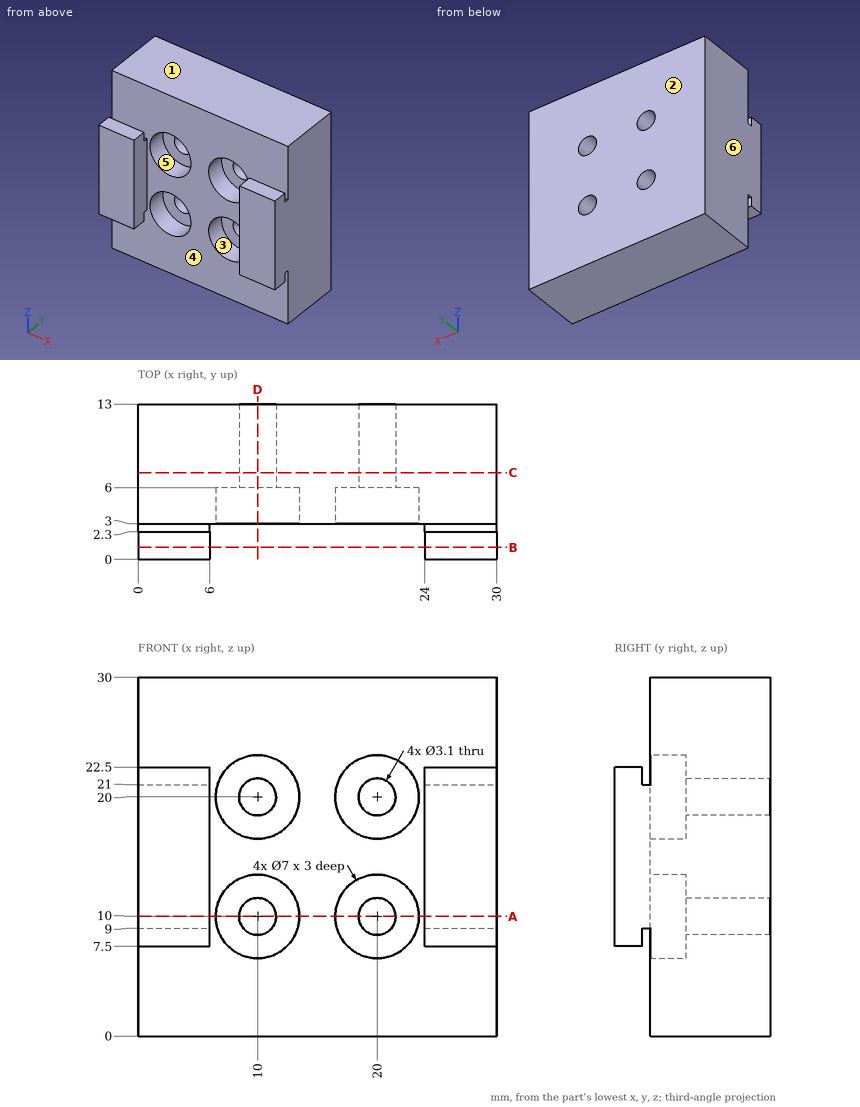
Answer from the drawing. Dimensions are ordinates in mm from the lowest x, y and z of the part. A direction names the side the tool comes from. Give positions to 0.01 mm unless a question says otherwise; leave off trailing zeros. Write each loop counter-clockwise with the first axis right and the second up, starting at its lowest first coordinate (ties: lowest second). Pieces come first, ordered by that corner, then holes. Notation, with made-up numbers: (78.5, 25.5) -> (85.5, 25.5) arc R9 ccw to (85.5, 30.5) -> close; hole circle Ø10 at (28, -18.75). An arc over 180 degrees is marked (long way). One line per question, with ' | ' between items. Start each with the question number.
1. Section C-C (y = 7.25) is taken. Determine the outline of the cut face in (x, z), plus the area to 3 significant figures.
2. For a pull along Z with two mould halves and no side action, classify the marked faces 1, 2 and 3 as pulls with the +Z half, pulls with the -Z half, needs draft (parallel to the pull), parting line crosses it, or undercut.
3. Section D-D (x = 10) is taken. Determine the outline of the cut face in (y, z), plus the area to 3 significant figures.
4. Find the intervals of material crossed by probe 1 along X at (y, z) = (4.55, 20); probe 2 along Z at (x, y) = (10, 9.75), in increasing order.
5. Given pin 1 Ø0.7 at (x, y) = (28, 1.5) entering from -Z; pin 2 Ø5.5 at (x, z) = (20.5, 9) entering from -Y; pin 3 Ø0.6 at (x, y) = (3.5, 2.5) entering from +Z, each flat-ended and moving along its own axis, determine where each tip first touches the part or whether it passes through.
6. For the marked faces 4, 5 and 6, determine the directions among +Z, -Z, +X, -X, +Y, -Y from which every point of the face is accessible in a straight line to the end or side of a thin tool.
7. Section A-A (z = 10) is taken. Determine the outline of the cut face in (x, y).
8. Section B-B (y = 1) is taken. Determine the outline of the cut face in (x, z).
Response values:
1) outline: (0, 0) -> (30, 0) -> (30, 30) -> (0, 30) -> close; hole circle Ø3.1 at (10, 10); hole circle Ø3.1 at (10, 20); hole circle Ø3.1 at (20, 10); hole circle Ø3.1 at (20, 20) | area: 870 mm2
2) face 1: pulls with the +Z half | face 2: needs draft | face 3: undercut
3) outline: (3, 0) -> (13, 0) -> (13, 8.45) -> (6, 8.45) -> (6, 6.5) -> (3, 6.5) -> close; (3, 13.5) -> (6, 13.5) -> (6, 11.55) -> (13, 11.55) -> (13, 18.45) -> (6, 18.45) -> (6, 16.5) -> (3, 16.5) -> close; (3, 23.5) -> (6, 23.5) -> (6, 21.55) -> (13, 21.55) -> (13, 30) -> (3, 30) -> close | area: 215 mm2
4) probe 1: 0 to 6.5, 13.5 to 16.5, 23.5 to 30 | probe 2: 0 to 8.45, 11.55 to 18.45, 21.55 to 30
5) pin 1: z = 7.5 | pin 2: y = 3 | pin 3: z = 22.5
6) face 4: none | face 5: -Y | face 6: +Z, -Z, -X, +Y, -Y
7) outline: (0, 0) -> (6, 0) -> (6, 3) -> (6.5, 3) -> (6.5, 6) -> (8.45, 6) -> (8.45, 13) -> (0, 13) -> close; (11.55, 6) -> (13.5, 6) -> (13.5, 3) -> (16.5, 3) -> (16.5, 6) -> (18.45, 6) -> (18.45, 13) -> (11.55, 13) -> close; (21.55, 6) -> (23.5, 6) -> (23.5, 3) -> (24, 3) -> (24, 0) -> (30, 0) -> (30, 13) -> (21.55, 13) -> close
8) outline: (0, 7.5) -> (6, 7.5) -> (6, 22.5) -> (0, 22.5) -> close; (24, 7.5) -> (30, 7.5) -> (30, 22.5) -> (24, 22.5) -> close
